Design review of the part shown in the three views and the two pictorial views. Dimensions are in mm from the part's minimum x, y and z. A direction names the side the tool comes from. Coordinates: 2 decimals unless noted, no trailing zeros. Loops run counter-clockwise (first coordinate to the right, second up) from the corner with the lowest first, then second, coordinate; pieces in that order, holes last. Notation, with made-up numbers: M 16.5,25.5 L 66.5,25.5 A18 cw 66.5,31.5 Z; hole C -14,9.5 d8. An arc over 180 degrees is marked long. Write item = value, one per line. Start each with the question number.
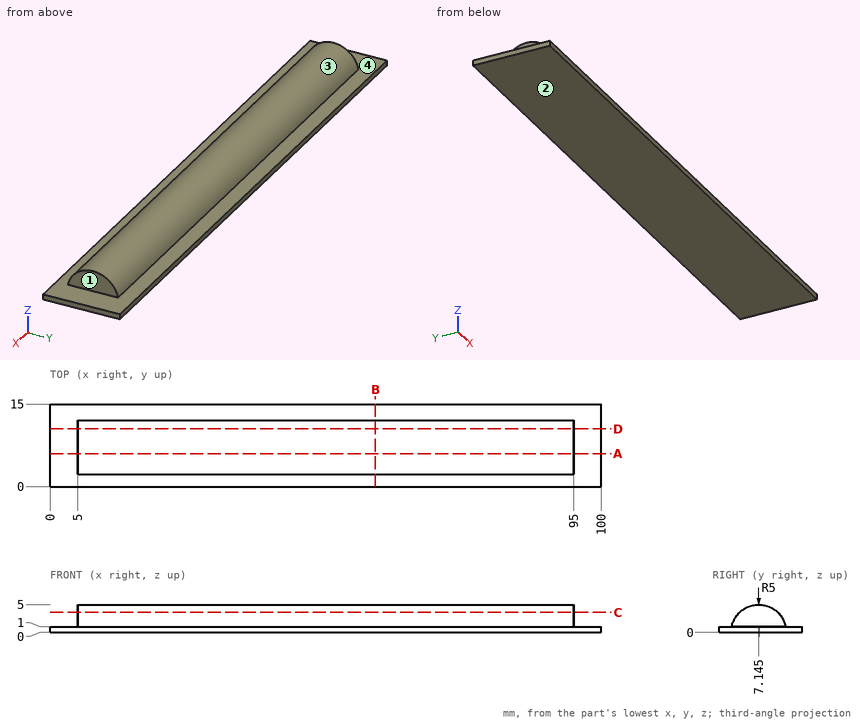
(1) Take a section at C-C (z = 3.6). State the section outline as (x, y) points (1 decimal).
(2) Take a section at B-B (x = 59). State the section outline as (y, z) points (1 decimal).
(3) Take a section at A-A (y = 6). State the section outline as (x, z) points.
(4) To check wall thickness, follow L1, parallel to X at y = 3.25, z = 1.55; L2, parallel to Z at x = 14.5, y = 1.75; L3, parallel to Z at x = 48, y = 7.25. State the ranges of each line that lie inside material, in increasing order.
(5) Tool access review of the marked faces 1 and 2: name each direction out of +Z, -Z, +X, -X, +Y, -Y from which nothing blocks a thin tool from reaching the whole face with its end or side.
(6) Insertion check: pin 1 (8 mm diameter, centred on x = 46.5, y = 9.5, fed in from -Z); pin 2 (1.2 mm diameter, centred on y = 5, z = 3, fed in from +X); pin 3 (3 mm diameter, centred on y = 10.5, z = 3, fed in from -X); pin 4 (1.5 mm diameter, centred on x = 47, z = 2, fed in from +Y) (1 decimal). Each pin has a flat end and moves straight along its axis. Give the tip position at first contact, or say it passes through.
(7) Mouldability with a two-part tool opening along Y and no side actions: class the marked faces 3 and 4 as +Y half, -Y half, draft (parallel to the pull), parting line (faces both ways), or undercut.
(8) Take a section at D-D (y = 10.5). State the section outline as (x, z) points.
Results list:
q1.outline = M 5,3.7 L 95,3.7 L 95,10.6 L 5,10.6 Z
q2.outline = M 0,0 L 15,0 L 15,1 L 12,1 A5 ccw 2.2,1 L 0,1 Z
q3.outline = M 0,0 L 100,0 L 100,1 L 95,1 L 95,4.87 L 5,4.87 L 5,1 L 0,1 Z
q4.L1 = 5 to 95
q4.L2 = 0 to 1
q4.L3 = 0 to 5
q5.face_1 = +Z, +X, +Y, -Y
q5.face_2 = -Z, +X, -X, +Y, -Y
q6.pin_1 = 0
q6.pin_2 = 95
q6.pin_3 = 5
q6.pin_4 = 12
q7.face_3 = parting line
q7.face_4 = draft
q8.outline = M 0,0 L 100,0 L 100,1 L 95,1 L 95,3.71 L 5,3.71 L 5,1 L 0,1 Z
